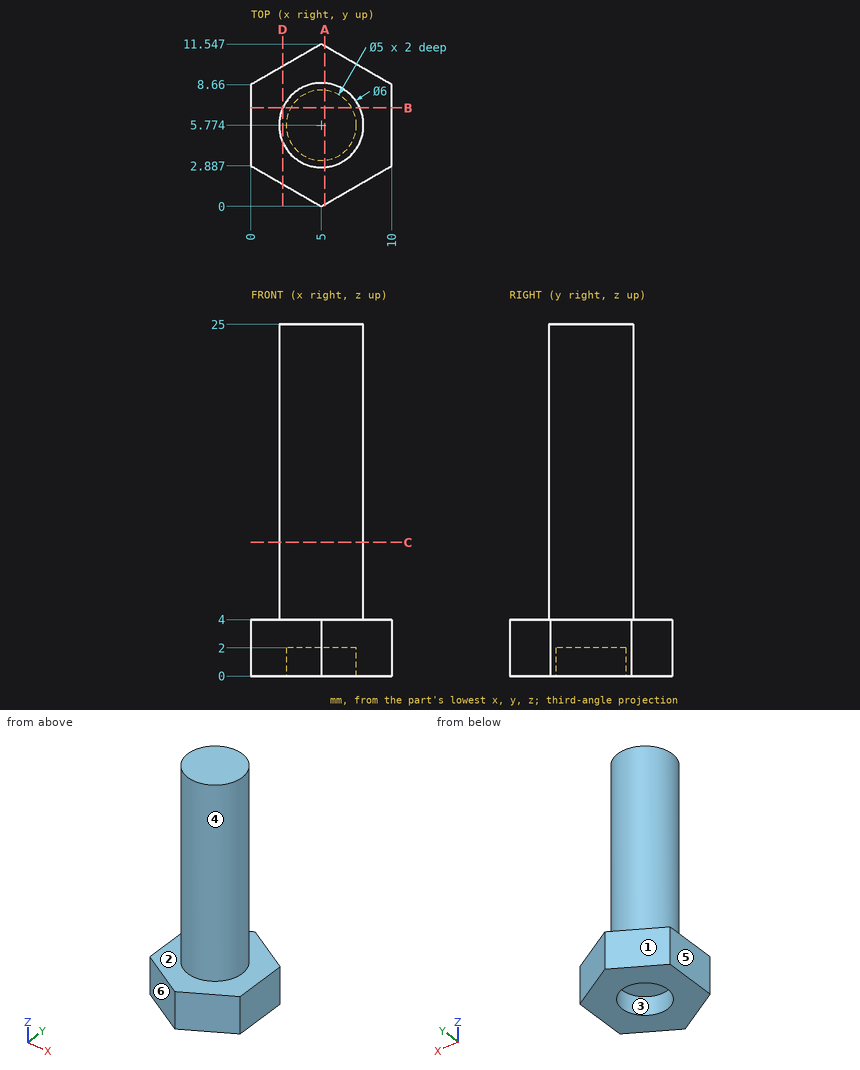
Verification items for this drawing (mm, ordinates from the low corner). A direction names the side the tool comes from. Give positions to 0.01 mm unless a question says otherwise; leave off trailing zeros. Order: outer loops, then holes, each group sorted by start corner. A loop starts at its lowest first (then second) coordinate and runs counter-clockwise, first axis right, second up. Notation, with made-up numbers: M -39.75,-36.5 L -30.75,-36.5 A19 ccw -30.75,-18.5 Z; hole C -1,89 d8. An arc over 180 degrees is marked long. Use a Markdown table: item, result.
Item 1: Material ranges on line 1 along Z through (x, y) = (5, 10.25); line 2 along Z through (x, y) = (5.5, 5.25); line 3 along Y through (x, z) = (3.75, 2.5) (1 decimal), recorded low to high.
Answers follow:
| item | result |
|---|---|
| line 1 | z = 0 to 4 |
| line 2 | z = 2 to 25 |
| line 3 | y = 0.7 to 10.8 |
Item 2: Tool access check on the marked faces 1 and 2. Record the directions out of +Z, -Z, +X, -X, +Y, -Y that give a thin tool (end or side, any length) a straight path to the whole face; none if there is none.
Answers follow:
| item | result |
|---|---|
| face 1 | +Z, -Z, -X, +Y |
| face 2 | +Z |
Item 3: Section check C-C (z = 9.5). Record the cut outline in (x, y), and give its area (3 significant figures).
Answers follow:
| item | result |
|---|---|
| outline | C 5,5.77 d6 |
| area | 28.3 mm2 |
Item 4: Section check B-B (y = 7). Record the cut outline in (x, z), and give its area (3 significant figures).
Answers follow:
| item | result |
|---|---|
| outline | M 0,0 L 2.82,0 L 2.82,2 L 7.18,2 L 7.18,0 L 10,0 L 10,4 L 7.74,4 L 7.74,25 L 2.26,25 L 2.26,4 L 0,4 Z |
| area | 146 mm2 |
Item 5: Draft check along Y on the marked faces 3, 4, 5 and 6. Enter one of: +Y half, -Y half, draft (parallel to the pull), parting line (faces both ways), or undercut.
Answers follow:
| item | result |
|---|---|
| face 3 | undercut |
| face 4 | parting line |
| face 5 | draft |
| face 6 | -Y half |
Item 6: Depth check by flat-ended pin: P1, Ø1.5, axis at x = 5, y = 9, coming from the +Z side; P2, Ø2, axis at x = 6, y = 6.5, coming from the -Z side. Enter the tip coordinate at first touch or a pass-through.
Answers follow:
| item | result |
|---|---|
| P1 | stops at z = 25 |
| P2 | stops at z = 2 |
Item 7: Section check A-A (x = 5.25). Record the cut outline in (y, z) (1 decimal), and give its area (3 significant figures).
Answers follow:
| item | result |
|---|---|
| outline | M 0.1,0 L 3.3,0 L 3.3,2 L 8.3,2 L 8.3,0 L 11.4,0 L 11.4,4 L 8.8,4 L 8.8,25 L 2.8,25 L 2.8,4 L 0.1,4 Z |
| area | 161 mm2 |
Item 8: Section check D-D (x = 2.25). Record the cut outline in (y, z) (1 decimal).
Answers follow:
| item | result |
|---|---|
| outline | M 1.6,0 L 10,0 L 10,4 L 7,4 L 7,25 L 4.6,25 L 4.6,4 L 1.6,4 Z |
